```python
from build123d import *

# Parameters (mm, degrees)
F0_W      = 8
F0_H      = 6.8
F1_DEPTH  = 1.5
F2_DEPTH  = 6.8
F4_DEPTH  = 1.5
F6_DEPTH  = 2
F7_W      = 9.5
F7_H      = 1.5
F8_DEPTH  = 2
F9_W      = 9.5
F9_H      = 1.5
F10_DEPTH = 2
F11_F1_R  = 1
F11_F2_R  = 1


with BuildPart() as f1:
    # F0 (on Top) → F1 (new body)
    with BuildSketch(Plane.XY):
        Polygon((4, 3.4), (4, -3.4), (-4, -3.4), (-4, -4.9), (5.5, -4.9), (5.5, 4.9), (-4, 4.9), (-4, 3.4), align=None)
        Rectangle(F0_W, F0_H)
    extrude(amount=-F1_DEPTH)

    # F0 (on Top) → F2 (join)
    with BuildSketch(Plane.XY):
        Polygon((4, 3.4), (4, -3.4), (-4, -3.4), (-4, -4.9), (5.5, -4.9), (5.5, 4.9), (-4, 4.9), (-4, 3.4), align=None)
    extrude(amount=F2_DEPTH)

    # F3 (on face) → F4 (join)
    with BuildSketch(Plane.XY.offset(6.8)):
        with BuildLine():
            ThreePointArc((0, 2.75), (2.75, 0), (0, -2.75))
            Line((0, -2.75), (-4, -2.75))
            Line((-4, -2.75), (-4, -3.4))
            Line((-4, -3.4), (4, -3.4))
            Line((4, -3.4), (4, 3.4))
            Line((4, 3.4), (-4, 3.4))
            Line((-4, 3.4), (-4, 2.75))
            Line((-4, 2.75), (0, 2.75))
        make_face()
        Polygon((4, -3.4), (-4, -3.4), (-4, -4.9), (5.5, -4.9), (5.5, 4.9), (-4, 4.9), (-4, 3.4), (4, 3.4), align=None)
    extrude(amount=F4_DEPTH)

    # F5 (on face) → F6 (join)
    with BuildSketch(Plane.XY.offset(8.3)):
        with BuildLine():
            ThreePointArc((0, 2.75), (2.75, 0), (0, -2.75))
            Line((0, -2.75), (-2.1650635095, -2.75))
            ThreePointArc((-2.1650635095, -2.75), (3.5, 0), (-2.1650635095, 2.75))
            Line((-2.1650635095, 2.75), (0, 2.75))
        make_face()
        with BuildLine():
            ThreePointArc((-1.3555844547, 2.3926744004), (-0.7009441486, 2.6591685356), (0, 2.75))
            Line((0, 2.75), (-2.1650635095, 2.75))
            ThreePointArc((-2.1650635095, 2.75), (-2.2741617405, 2.6604864928), (-2.3795628172, 2.5666477747))
            ThreePointArc((-2.3795628172, 2.5666477747), (-2.4155229026, 2.507985001), (-2.4157537689, 2.4391780576))
            ThreePointArc((-2.4157537689, 2.4391780576), (-1.8923464861, 2.2636984741), (-1.3555844547, 2.3926744004))
        make_face()
        with BuildLine():
            ThreePointArc((0, -2.75), (-0.7009441486, -2.6591685356), (-1.3555844547, -2.3926744004))
            ThreePointArc((-1.3555844547, -2.3926744004), (-1.8923464861, -2.2636984741), (-2.4157537689, -2.4391780576))
            ThreePointArc((-2.4157537689, -2.4391780576), (-2.4155229026, -2.507985001), (-2.3795628172, -2.5666477747))
            ThreePointArc((-2.3795628172, -2.5666477747), (-2.2741617405, -2.6604864928), (-2.1650635095, -2.75))
            Line((-2.1650635095, -2.75), (0, -2.75))
        make_face()
    extrude(amount=F6_DEPTH)

    # F7 (on face) → F8 (join)
    with BuildSketch(Plane(origin=(0, 4.9, 0), x_dir=(-1, 0, 0), z_dir=(0, 1, 0))):
        with Locations((-0.75, 7.55)):
            Rectangle(F7_W, F7_H)
    extrude(amount=F8_DEPTH)

    # F9 (on face) → F10 (join)
    with BuildSketch(Plane.XZ.offset(4.9)):
        with Locations((0.75, 7.55)):
            Rectangle(F9_W, F9_H)
    extrude(amount=F10_DEPTH)

    # F11: fillet of radius 1 on 16 edges, made by hand

    # F11_f1
    f11_f1_edges = [f1.edges().sort_by_distance(p)[0] for p in [
        (0.75, -4.9, 6.8),
        (0.75, 4.9, 6.8),
    ]]
    fillet(f11_f1_edges, radius=F11_F1_R)

    # F11_f2
    f11_f2_edges = [f1.edges().sort_by_distance(p)[0] for p in [
        (0.75, -4.9, -1.5),
        (5.5, -4.9, 2.15),
        (5.5, 4.9, 2.15),
        (5.5, 0, -1.5),
        (0.75, 4.9, -1.5),
        (-4, 4.9, 2.15),
        (-4, 0, -1.5),
        (-4, -4.9, 2.15),
        (-4, 6.9, 7.55),
        (-4, 6.4, 6.8),
        (5.5, 6.9, 7.55),
        (5.5, -6.9, 7.55),
        (-4, -6.9, 7.55),
        (-4, -6.4, 6.8),
        (-4, -5.1928932188, 6.5071067812),
        (-4, 5.1928932188, 6.5071067812),
        (5.5, 5.1928932188, 6.5071067812),
        (5.5, -5.1928932188, 6.5071067812),
    ]]
    fillet(f11_f2_edges, radius=F11_F2_R)


solid = f1.part
```
The listing builds one solid part. Answer for the finished solid, in the listing's coordinates (mm). A direction names the side the tool comes from. Coordinates: 2 decimals unless noted, no trailing zeros. Write each loop counter-clockwise with the first axis right and the second up, starting at its lowest first coordinate (ties: lowest second). Pieces come first, ordered by that corner, then holes. Notation, with made-up numbers: M 35.25,57 L 44.25,57 A38 cw 44.25,95 Z; hole C -8,35 d4. An arc over 180 degrees is marked long. Use a Markdown table: item, result. Add a question column.
1. Given P1, Ø2, axis at y = 5, z = 6, coming from the -X side; P2, Ø2, axis at x = -3, z = 9, coming from the +Y side; P3, Ø1, axis at x = 0, z = 1, coming from the +Y side; P4, Ø5, axis at x = 2, z = 4, coming from the -Y side, each flat-ended and moving along its own axis, determine where each tip first touches the part or whether it passes through.
2. Section D-D (z = 9.25) is taken. Give the vertices of the cut face in (x, y), plus the area to 3 significant figures.
3. Which of the six approach directions +Z, -Z, +X, -X, +Y, -Y give full straight-line access (tool end or side, diameter ignored) to faces 4 (the flat face through (0.8, 6.4, 6.8)), 5 (the cylindrical face through (5.1, 6.3, 7)), 6 (the cylindrical face through (-3.715, 4.599, 2.606)), 7 (the cylindrical face through (5.1, -6.3, 7)), 8 (the cylindrical face through (-1.9, 2.264, 9.286))?
4. Section B-B (y = 0) is taken. Give the vertices of the cut face in (x, z).
5. Section C-C (x = 1.25) is taken. Give the vertices of the cut face in (y, z).
6. Straight lines are drawn through the part: line 1 along Z through (x, y) = (2, -2.5); line 2 along Z through (x, y) = (1.5, 3.25); line 3 along Y through (x, z) = (-0.25, 5). For each, find the intervals that lie inside material, in ascending order. Write a range as [from, to].
7. For a pull along Y with two mould halves and no side action, classify faces 1 (the flat face through (4, 0, 3)), 2 (the flat face through (1, -6.9, 8)), 3 (the cylindrical face through (5.199, 4.615, 2.694)) as +Y half, -Y half, draft (parallel to the pull), parting line (faces both ways), or undercut.
8. Section A-A (z = 2.5) is taken. Give the vertices of the cut face in (x, y), plus the area to 3 significant figures.
Data:
| question | item | result |
|---|---|---|
| 1 | P1 | stops at x = -4 |
| 1 | P2 | stops at y = 6.9 |
| 1 | P3 | stops at y = 4.9 |
| 1 | P4 | stops at y = -5.19 |
| 2 | outline | M -2.42,-2.44 A0.13 ccw -2.38,-2.57 A3.5 ccw long -2.38,2.57 A0.13 ccw -2.42,2.44 A1 ccw -1.36,2.39 A2.75 cw long -1.36,-2.39 A1 ccw Z |
| 2 | area | 10.8 mm2 |
| 3 | face 4 | -Z, +X, -X, +Y |
| 3 | face 5 | -Z, +X, +Y |
| 3 | face 6 | -Z, -X, +Y |
| 3 | face 7 | -Z, +X, -Y |
| 3 | face 8 | +Z |
| 4 | outline | M -4,-0.5 A1 ccw -3,-1.5 L 4.5,-1.5 A1 ccw 5.5,-0.5 L 5.5,8.3 L 3.5,8.3 L 3.5,10.3 L 2.75,10.3 L 2.75,6.8 L 4,6.8 L 4,0 L -4,0 Z |
| 5 | outline | M -6.9,6.8 L -5.9,6.8 A1 cw -4.9,5.8 L -4.9,-0.5 A1 ccw -3.9,-1.5 L 3.9,-1.5 A1 ccw 4.9,-0.5 L 4.9,5.8 A1 cw 5.9,6.8 L 6.9,6.8 L 6.9,8.3 L 3.27,8.3 L 3.27,10.3 L 2.45,10.3 L 2.45,6.8 L 3.4,6.8 L 3.4,0 L -3.4,0 L -3.4,6.8 L -2.45,6.8 L -2.45,10.3 L -3.27,10.3 L -3.27,8.3 L -6.9,8.3 Z |
| 6 | line 1 | z = [-1.5, 0], [6.8, 10.3] |
| 6 | line 2 | z = [-1.5, 0], [6.8, 8.3] |
| 6 | line 3 | y = [-4.9, -3.4], [3.4, 4.9] |
| 7 | face 1 | undercut |
| 7 | face 2 | -Y half |
| 7 | face 3 | +Y half |
| 8 | outline | M -4,-3.9 A1 ccw -3,-4.9 L 4.5,-4.9 A1 ccw 5.5,-3.9 L 5.5,3.9 A1 ccw 4.5,4.9 L -3,4.9 A1 ccw -4,3.9 L -4,3.4 L 4,3.4 L 4,-3.4 L -4,-3.4 Z |
| 8 | area | 37.8 mm2 |
